Answer from the drawing. Dimensions are ordinates in mm from the lowest x, y and z of the part. Round coordinates to 2 decimals unless told otherwise and drop trailing zeros. Write each loop counter-clockwise with the first axis right and the second up, starting at its lowest first coordinate (ties: lowest second). Pieces come first, ordered by that corner, then holes. Notation, with made-up numbers: M -18.75,78 L 27.25,78 A13 cw 27.25,101 Z; hole C 13.5,-14.75 d3. An arc over 180 degrees is marked long. One line per item, written item: value. Start each with the question number.
(1) Section A-A (x = 19.95) is taken. Determine the outline of the cut face in (y, z), plus the area to 3 significant figures.
(2) Section B-B (y = 4.5) is taken. Determine the outline of the cut face in (x, z), plus the area to 3 significant figures.
(3) Given P1, Ø2, axis at y = 3.5, z = 7.5, coming from the +X side, flat-ended and moving along its own axis, determine where the tip first touches the part or whether it passes through.
(4) For a pull along X with two mould halves and no side action, classify the marked faces 1 and 2 as released by +X, released by -X, zero draft, split by the parting line, or undercut.
(5) Section C-C (z = 7.5) is taken. Determine the outline of the cut face in (x, y).
(6) Section D-D (x = 27.65) is taken. Determine the outline of the cut face in (y, z), plus the area to 3 significant figures.
(7) Consider probe 1 along Z at (x, y) = (3.25, 3.5); probe 2 along Z at (x, y) = (10.95, 6.25); probe 3 along X at (y, z) = (5.75, 7.75). Determine where each line is inside the solid, lowest interval first.
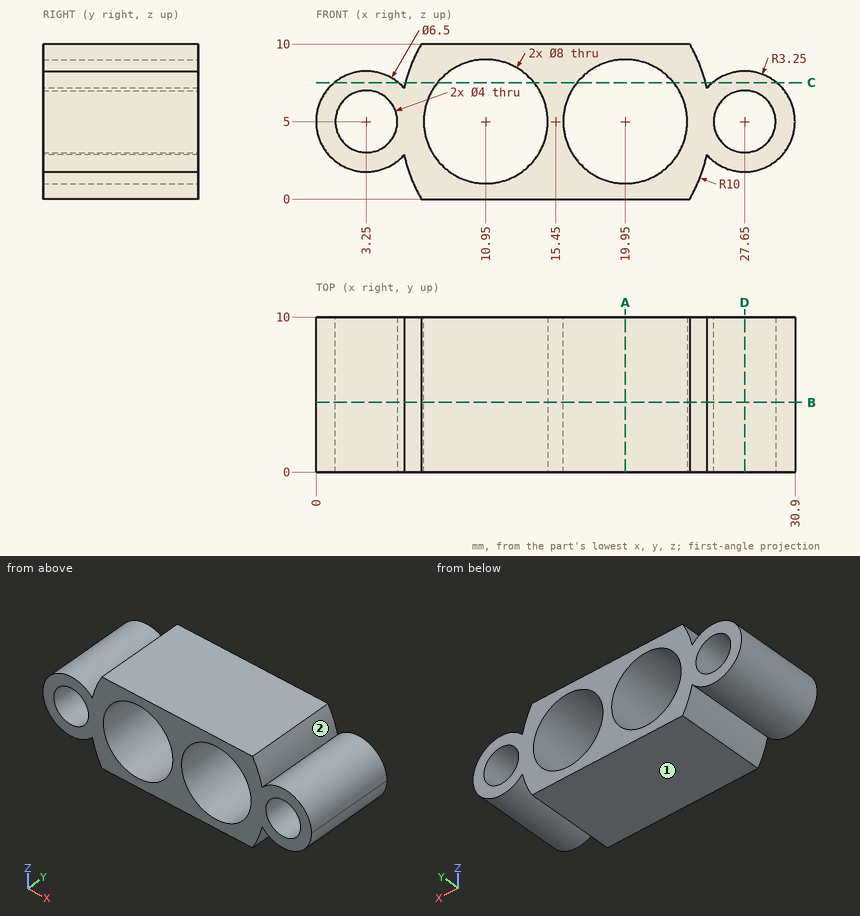
Recorded:
1. outline: M 0,0 L 10,0 L 10,1 L 0,1 Z; M 0,9 L 10,9 L 10,10 L 0,10 Z
1. area: 20.0 mm2
2. outline: M 5.68,2.85 A10 ccw 6.79,0 L 24.11,0 A10 ccw 25.22,2.85 A3.25 ccw long 25.22,7.15 A10 ccw 24.11,10 L 6.79,10 A10 ccw 5.68,7.15 A3.25 ccw long Z; hole C 3.25,5 d4; hole C 10.95,5 d8; hole C 19.95,5 d8; hole C 27.65,5 d4
2. area: 126 mm2
3. P1: stops at x = 30.53
4. face 1: zero draft
4. face 2: undercut
5. outline: M 1.17,0 L 5.33,0 L 5.33,10 L 1.17,10 Z; M 5.77,0 L 7.83,0 L 7.83,10 L 5.77,10 Z; M 14.07,0 L 16.83,0 L 16.83,10 L 14.07,10 Z; M 23.07,0 L 25.13,0 L 25.13,10 L 23.07,10 Z; M 25.57,0 L 29.73,0 L 29.73,10 L 25.57,10 Z
6. outline: M 0,1.75 L 10,1.75 L 10,3 L 0,3 Z; M 0,7 L 10,7 L 10,8.25 L 0,8.25 Z
6. area: 25.0 mm2
7. probe 1: z = 1.75 to 3, 7 to 8.25
7. probe 2: z = 0 to 1, 9 to 10
7. probe 3: x = 1.52 to 4.98, 5.84 to 8.05, 13.85 to 17.05, 22.85 to 25.06, 25.92 to 29.38
